Autodesk Inventor part; units mm, degrees
ref_plane "YZ Plane" through (0, 0, 0) normal (1, 0, 0) x (0, 1, 0)
ref_plane "XZ Plane" through (0, 0, 0) normal (0, 1, 0) x (-1, 0, 0)
ref_plane "XY Plane" through (0, 0, 0) normal (0, 0, 1) x (1, 0, 0)
sketch "Sketch1" plane through (0, 0, 0) normal (0, 0, 1) x (1, 0, 0)
  line L0 (0, 0) -> (20, 0)
  line L1 (20, 0) -> (20, 30)
  line L2 (20, 30) -> (0, 30)
  line L3 (0, 30) -> (0, 0)
  dimension "d0" = 20
  dimension "d1" = 30
extrude "Extrusion1" add sketch "Sketch1" along normal blind 10
fillet "Fillet1" radius 2 4 edges at (0, 15, 10) (20, 15, 10) (20, 15, 0) (0, 15, 0)
sketch "Sketch2" plane through (2, 30, 0) normal (0, 1, 0) x (1, 0, 0)
  line L0 (15.25, -2.5) -> (0.75, -2.5)
  line L1 (0.75, -2.5) -> (0.75, -5.5)
  line L2 (15.25, -2.5) -> (15.25, -5.5)
  line L3 (13, -7.5) -> (3, -7.5)
  line L4 (16, -10) -> (0, -10)
  line L5 (8, -2.5) -> (8, -7.5) construction
  line L6 (18, -2) -> (18, -8)
  arc A0 (15.25, -5.5) -> (13, -7.5) centre (16.5871, -9.2699) ccw
  arc A1 (3, -7.5) -> (0.75, -5.5) centre (-0.5871, -9.2699) ccw
  point P0 (-2, 0)
  point P1 (8, -10)
  point P2 (8, -5)
  point P3 (18, -5)
  dimension "d5" = 14.5
  dimension "d6" = 3
  dimension "d7" = 2
  dimension "d8" = 10
  dimension "d9" = 4
  dimension "d10" = 4
extrude "Extrusion2" cut sketch "Sketch2" against normal blind 10
sketch "Sketch3" plane through (2, 20, 0) normal (0, 1, 0) x (1, 0, 0)
  line L0 (0.75, -2.5) -> (15.25, -2.5)
  line L1 (0.75, -5.5) -> (0.75, -2.5)
  arc A0 (3, -7.5) -> (0.75, -5.5) centre (-0.5871, -9.2699) ccw
  line L2 (13, -7.5) -> (3, -7.5)
  arc A1 (15.25, -5.5) -> (13, -7.5) centre (16.5871, -9.2699) ccw
  line L3 (15.25, -2.5) -> (15.25, -5.5)
  arc A2 (2.8734, -7.7) -> (0.55, -5.644) centre (-0.5871, -9.2699) ccw
  line L4 (0.55, -5.644) -> (0.55, -2.3)
  line L5 (0.55, -2.3) -> (15.45, -2.3)
  line L6 (15.45, -2.3) -> (15.45, -5.644)
  arc A3 (15.45, -5.644) -> (13.1266, -7.7) centre (16.5871, -9.2699) ccw
  line L7 (13.1266, -7.7) -> (2.8734, -7.7)
  point P0 (-2, 0)
  dimension "d13" = 0.2
extrude "Extrusion3" add sketch "Sketch3" along normal blind 10.1
sketch "Sketch4" plane through (2, 20, 0) normal (0, 1, 0) x (1, 0, 0)
  line L0 (13.5, -5) -> (2.5, -5)
  line L1 (2.5, -5) -> (2.5, -4)
  line L2 (2.5, -4) -> (13.5, -4)
  line L3 (13.5, -4) -> (13.5, -5)
  line L4 (13, -7.5) -> (3, -7.5)
  line L5 (0.75, -2.5) -> (15.25, -2.5)
  point P0 (-2, 0)
  point P1 (8, -5)
  point P2 (8, -7.5)
  dimension "d16" = 11
  dimension "d17" = 1
  dimension "d18" = 1.5
extrude "Extrusion4" add sketch "Sketch4" along normal blind 8
properties part number "HDMI Port" material "ABS Plastic"
Read the model definition and answer for the solid it produces. Units are mm, in the model's axes. A direction names the side the tool comes from. Coordinates: 2 decimals unless noted, no trailing zeros. Write each loop counter-clockwise with the first axis right and the second up, starting at its lowest first coordinate (ties: lowest second). Pieces come first, ordered by that corner, then holes. Notation, with made-up numbers: (-21, 17.25) -> (38, 17.25) arc R13 cw to (38, 40.25) -> close; hole circle Ø8 at (-28, -5.5). An arc over 180 degrees is marked (long way). Return JSON: item names as keys, results as strings.
(1) The part is cut by section A-A on y = 24.5. Give the vertices of the cut face in (x, z).
Answers below:
{"outline": "(0, 2) arc R2 ccw to (2, 0) -> (18, 0) arc R2 ccw to (20, 2) -> (20, 8) arc R2 ccw to (18, 10) -> (2, 10) arc R2 ccw to (0, 8) -> close; (4.5, 4) -> (15.5, 4) -> (15.5, 5) -> (4.5, 5) -> close; hole (2.75, 2.5) -> (17.25, 2.5) -> (17.25, 5.5) arc R4 cw to (15, 7.5) -> (5, 7.5) arc R4 cw to (2.75, 5.5) -> close"}
(2) The part is cut by section D-D on y = 13.5. Give the vertices of the cut face in (x, z), then the cut area to 3 significant figures.
Answers below:
{"outline": "(0, 2) arc R2 ccw to (2, 0) -> (18, 0) arc R2 ccw to (20, 2) -> (20, 8) arc R2 ccw to (18, 10) -> (2, 10) arc R2 ccw to (0, 8) -> close", "area": "197 mm^2"}
(3) Consider line 1 along X through (y, z) = (22.5, 4.5); line 2 along Z through (x, y) = (14.5, 21.5); line 3 along Z through (x, y) = (3.75, 25.5). Determine where each line is inside the solid, lowest interval first. Write a range as from..to.
Answers below:
{"line 1": "0..2.75, 4.5..15.5, 17.25..20", "line 2": "0..2.5, 4..5, 7.5..10", "line 3": "0..2.5, 6.02..10"}
(4) For a pull along Z with two mould halves and no side action, classify faces 1 (the flat face through (0, 15, 5)), 2 (the flat face through (10, 15, 0)), 3 (the flat face through (10, 15, 10)), 4 (the flat face through (4.5, 23.9, 4.5)) as pulls with the +Z half, pulls with the -Z half, needs draft (parallel to the pull), parting line crosses it, or undercut.
Answers below:
{"face 1": "needs draft", "face 2": "pulls with the -Z half", "face 3": "pulls with the +Z half", "face 4": "undercut"}
(5) Which of the six approach directions +Z, -Z, +X, -X, +Y, -Y give full straight-line access (tool end or side, diameter ignored) to faces 5 (the flat face through (10, 0, 5)), 6 (the flat face through (10, 24, 5))?
Answers below:
{"face 5": "+Z, -Z, +X, -X, -Y", "face 6": "+Y"}
(6) This flat-tipped pin is pushed along its axis until it touches: P1, Ø1.1, axis at x = 11.5, z = 4.5, coming from the +Y side. Where does it stop, or does it pass through?
Answers below:
{"P1": "y = 28"}
(7) The part is cut by section C-C on x = 9.25. Give the vertices of the cut face in (y, z), then the cut area to 3 significant figures.
Answers below:
{"outline": "(0, 0) -> (30, 0) -> (30, 2.3) -> (30.1, 2.3) -> (30.1, 2.5) -> (20, 2.5) -> (20, 4) -> (28, 4) -> (28, 5) -> (20, 5) -> (20, 7.5) -> (30.1, 7.5) -> (30.1, 7.7) -> (30, 7.7) -> (30, 10) -> (0, 10) -> close", "area": "258 mm^2"}
(8) The part is cut by section B-B on z = 4.5. Give the vertices of the cut face in (x, y), then the cut area to 3 significant figures.
Answers below:
{"outline": "(0, 0) -> (20, 0) -> (20, 30) -> (17.45, 30) -> (17.45, 30.1) -> (17.25, 30.1) -> (17.25, 20) -> (15.5, 20) -> (15.5, 28) -> (4.5, 28) -> (4.5, 20) -> (2.75, 20) -> (2.75, 30.1) -> (2.55, 30.1) -> (2.55, 30) -> (0, 30) -> close", "area": "543 mm^2"}
